```python
from build123d import *

# Parameters (mm, degrees)
BOSS_EXTRUDE1_DEPTH = 1.5875
SKETCH2_W           = 6.35
SKETCH2_H           = 6.35
BOSS_EXTRUDE3_DEPTH = 6.35
SKETCH2_4_R         = 2.54
BOSS_EXTRUDE4_DEPTH = 12.7
BOSS_EXTRUDE4_TAPER = 1.5
CHAMFER1_SIZE       = 1.27


with BuildPart() as part:
    # Sketch1 → Boss-Extrude1 (new body)
    with BuildSketch(Plane.XY):
        with BuildLine():
            Line((-10.16, 12.7), (10.16, 12.7))
            ThreePointArc((10.16, 12.7), (11.956051224, 11.956051224), (12.7, 10.16))
            Line((12.7, 10.16), (12.7, -10.16))
            ThreePointArc((12.7, -10.16), (11.956051224, -11.956051224), (10.16, -12.7))
            Line((10.16, -12.7), (-10.16, -12.7))
            ThreePointArc((-10.16, -12.7), (-11.956051224, -11.956051224), (-12.7, -10.16))
            Line((-12.7, -10.16), (-12.7, 10.16))
            ThreePointArc((-12.7, 10.16), (-11.956051224, 11.956051224), (-10.16, 12.7))
        make_face()
    extrude(amount=BOSS_EXTRUDE1_DEPTH)

    # Sketch2 → Boss-Extrude3 (add)
    with BuildSketch(Plane.XY.offset(1.5875)):
        with Locations((0, -9.525)):
            Rectangle(SKETCH2_W, SKETCH2_H)
        with Locations((-9.525, 0)):
            Rectangle(SKETCH2_W, SKETCH2_H)
        with Locations((0, 9.525)):
            Rectangle(SKETCH2_W, SKETCH2_H)
    extrude(amount=BOSS_EXTRUDE3_DEPTH)

    # Sketch2<4> → Boss-Extrude4 (add)
    with BuildSketch(Plane.XY.offset(1.5875)):
        Circle(SKETCH2_4_R)
    extrude(amount=BOSS_EXTRUDE4_DEPTH, taper=BOSS_EXTRUDE4_TAPER)

    # Chamfer1
    chamfer1_edges = [part.edges().sort_by_distance(p)[0] for p in [
        (3.175, -9.525, 7.9375),
        (0, -6.35, 7.9375),
        (-3.175, -9.525, 7.9375),
        (-6.35, 0, 7.9375),
        (-9.525, 3.175, 7.9375),
        (-9.525, -3.175, 7.9375),
        (-3.175, 9.525, 7.9375),
        (0, 6.35, 7.9375),
        (3.175, 9.525, 7.9375),
    ]]
    chamfer(chamfer1_edges, length=CHAMFER1_SIZE)


solid = part.part
```
Can you work these out from the model? Positions are in its coordinate system, mm. A direction names the side the tool comes from. Round coordinates to 2 decimals unless told otherwise and drop trailing zeros. Loops run counter-clockwise (first coordinate to the right, second up) from the corner with the lowest first, then second, coordinate; pieces in that order, holes last. Notation, with made-up numbers: (-12, -13) -> (31, -13) arc R17 ccw to (31, -2) -> close; hole circle Ø5 at (85.5, -40). An arc over 180 degrees is marked (long way). Answer in a Markdown table with one row per item.
Item 1: Suppose I cut it at D-D, the plane z = 7.25. List the corners of the cut face in (x, y) for me.
Answer block:
| item | result |
|---|---|
| outline | (-12.7, -2.59) -> (-6.93, -2.59) -> (-6.93, 2.59) -> (-12.7, 2.59) -> close; (-2.59, -12.7) -> (2.59, -12.7) -> (2.59, -6.93) -> (-2.59, -6.93) -> close; (-2.59, 6.93) -> (2.59, 6.93) -> (2.59, 12.7) -> (-2.59, 12.7) -> close; circle Ø4.78 at (0, 0) |
Item 2: If I drill on probe 1 along Y at (x, z) = (-1.75, 2); probe 2 along Z at (x, y) = (0.5, 8.75); probe 3 along Y at (x, z) = (-0.75, 4.75), over which ranges is the centre line in solid material (lowest first)?
Answer block:
| item | result |
|---|---|
| probe 1 | -12.7 to -6.35, -1.83 to 1.83, 6.35 to 12.7 |
| probe 2 | 0 to 7.94 |
| probe 3 | -12.7 to -6.35, -2.34 to 2.34, 6.35 to 12.7 |
Item 3: Suppose I cut it at B-B, the plane x = 0. List the corners of the cut face in (y, z) for me, plus the area to 3 significant figures.
Answer block:
| item | result |
|---|---|
| outline | (-12.7, 0) -> (12.7, 0) -> (12.7, 7.94) -> (7.62, 7.94) -> (6.35, 6.67) -> (6.35, 1.59) -> (2.54, 1.59) -> (2.21, 14.29) -> (-2.21, 14.29) -> (-2.54, 1.59) -> (-6.35, 1.59) -> (-6.35, 6.67) -> (-7.62, 7.94) -> (-12.7, 7.94) -> close |
| area | 180 mm² |
Item 4: On a 3-axis mill with a long thin cutter (end or side, diameter ignored), from which of +Z, -Z, +X, -X, +Y, -Y can I reach the whole of each face in a straight line? I mean faces 5 (the flat face through (-3.175, -10, 4)), 6 (the flat face through (3.175, -10, 4)), 7 (the flat face through (-0.044, 6.976, 7.294)), 8 (the flat face through (-6.99, -0.04, 7.31)), 9 (the flat face through (0, 10, 7.938)). Say none if no direction works.
Answer block:
| item | result |
|---|---|
| face 5 | +Z, -X, +Y, -Y |
| face 6 | +Z, +X, +Y, -Y |
| face 7 | +Z, +X, -X |
| face 8 | +Z, +Y, -Y |
| face 9 | +Z, +X, -X, +Y |
Item 5: Suppose I cut it at C-C, the plane y = -9.25. List the corners of the cut face in (x, z) for me (1 decimal).
Answer block:
| item | result |
|---|---|
| outline | (-12.7, 0) -> (12.7, 0) -> (12.7, 1.6) -> (3.2, 1.6) -> (3.2, 6.7) -> (1.9, 7.9) -> (-1.9, 7.9) -> (-3.2, 6.7) -> (-3.2, 1.6) -> (-12.7, 1.6) -> close |
Item 6: Will these pins go through, and if not, where does the flat tip stop? P1, Ø2, axis at x = 8, z = 2.5, coming from the +Y side; P2, Ø4, axis at x = -9.5, y = 1, coming from the +Z side; P3, Ø4, axis at y = 8.5, z = 5, coming from the +X side (3 decimals); P4, Ø2.5, axis at y = -10.5, z = 3, coming from the -X side (3 decimals).
Answer block:
| item | result |
|---|---|
| P1 | y = 12.7 |
| P2 | z = 7.94 |
| P3 | x = 3.175 |
| P4 | x = -3.175 |
Item 7: Suppose I cut it at A-A, the plane z = 2. List the corners of the cut face in (x, y) for me (3 decimals), plus the area to 3 significant figures.
Answer block:
| item | result |
|---|---|
| outline | (-12.7, -3.175) -> (-6.35, -3.175) -> (-6.35, 3.175) -> (-12.7, 3.175) -> close; (-3.175, -12.7) -> (3.175, -12.7) -> (3.175, -6.35) -> (-3.175, -6.35) -> close; (-3.175, 6.35) -> (3.175, 6.35) -> (3.175, 12.7) -> (-3.175, 12.7) -> close; circle Ø5.058 at (0, 0) |
| area | 141 mm² |
Item 8: We'd pull the mould along X, two halves only. Please class faces 1 (the flat face through (-12.7, 0, 3)), 2 (the flat face through (2.55, 9.48, 7.29)), 3 (the flat face through (-9.57, 2.53, 7.31)), 4 (the flat face through (-6.35, 0, 4)): released by +X, released by -X, zero draft, split by the parting line, or undercut.
Answer block:
| item | result |
|---|---|
| face 1 | released by -X |
| face 2 | released by +X |
| face 3 | zero draft |
| face 4 | undercut |
